from build123d import *


with BuildPart() as part:
    # Sketch1 → Revolve1 (revolve)
    with BuildSketch(Plane(origin=(0, 0, 0), x_dir=(0, 0, -1), z_dir=(1, 0, 0))):
        with BuildLine():
            Line((-10.35, -0.083114039), (-10.35, 2.416885961))
            add(Edge.make_bspline(
                [(-10.35, 2.416885961), (-10.35, 3.365522707), (-5.87405228, 4.241080394), (-2.867984372, 4.033812591), (-2.611626956, 4.324223727), (-2.731131844, 4.758475996), (-2.197387439, 5.360223564), (-0.492736408, 5.316885961), (0, 5.316885961)],
                knots=[0, 0, 0, 0, 0.734908426, 0.759492363, 0.786959078, 0.823764272, 0.867168962, 1, 1, 1, 1], degree=3))
            Line((0, 5.316885961), (0, 3.882124351))
            Line((0, 3.882124351), (-1.400856338, 3.882124351))
            Line((-1.400856338, 3.882124351), (-1.400856338, 2.565845829))
            Line((-1.400856338, 2.565845829), (-6.683387829, 1.648087396))
            Line((-6.683387829, 1.648087396), (-6.683387829, -4.921019872))
            Line((-6.683387829, -4.921019872), (-3.287892009, -7.171193847))
            Line((-3.287892009, -7.171193847), (-3.759677095, -7.883114039))
            Line((-3.759677095, -7.883114039), (-7.30583237, -5.533098981))
            Line((-7.30583237, -5.533098981), (-7.30583237, -7.883114039))
            Line((-7.30583237, -7.883114039), (-8.159470598, -7.883114039))
            Line((-8.159470598, -7.883114039), (-8.159470598, -7.762098691))
            Line((-8.159470598, -7.762098691), (-9.5, -4.383114039))
            Line((-9.5, -4.383114039), (-9.5, -2.883114039))
            Line((-9.5, -2.883114039), (-8, -2.883114039))
            Line((-8, -2.883114039), (-8, -2.583114039))
            Line((-8, -2.583114039), (-8.366666667, -2.216447373))
            Line((-8.366666667, -2.216447373), (-8, -1.849780706))
            Line((-8, -1.849780706), (-8.366666667, -1.483114039))
            Line((-8.366666667, -1.483114039), (-8, -1.116447373))
            Line((-8, -1.116447373), (-8.366666667, -0.749780706))
            Line((-8.366666667, -0.749780706), (-8, -0.383114039))
            Line((-8, -0.383114039), (-8, -0.083114039))
            Line((-8, -0.083114039), (-10.35, -0.083114039))
        make_face()
    revolve(axis=Axis((0, 6.890935363, 0), (0, -1, 0)))


solid = part.part
CAD build for the part. Positions are in the model's coordinates, mm. A direction names the side the tool comes from. Round coordinates to 2 decimals unless told otherwise and drop trailing zeros. Order: outer loops, then holes, each group sorted by start corner. A loop starts at its lowest first (then second) coordinate and runs counter-clockwise, first axis right, second up. Notation, with made-up numbers: (89.25, 38.25) -> (115.25, 38.25) arc R16 ccw to (115.25, 48.25) -> close; hole circle Ø10 at (22.25, -22). An arc over 180 degrees is marked (long way). Write each question's results on one line, items separated by ' | '.
1. Wall check: line 1 along Z through (x, y) = (0, -5.95); line 2 along X through (y, z) = (-6.8, 0); line 3 along X through (y, z) = (0.5, 0). Give the ranges that are in metal, low to high. Write a range as [from, to].
Findings below:
line 1: z = [-8.88, -7.31], [-6.68, -5.13], [5.13, 6.68], [7.31, 8.88] | line 2: x = [-8.54, -7.31], [-5.39, -3.85], [3.85, 5.39], [7.31, 8.54] | line 3: x = [-10.35, -6.68], [6.68, 10.35]
2. Cut at A-A (y = -6.75). Give the cut face in (x, z).
Findings below:
outline: circle Ø17.12 at (0, 0); circle Ø10.94 at (0, 0); hole circle Ø14.61 at (0, 0); hole circle Ø7.85 at (0, 0)
3. Flat gauge pins, fed straight in: P1, Ø5, axis at x = 1.5, z = -3.5, coming from the +Y side; P2, Ø5, axis at y = 0, z = 5, coming from the -X side; P3, Ø5.5, axis at x = 4, z = 2, coming from the +Y side. Where does each tip first touch, or does it go through?
Findings below:
P1: stops at y = 5.29 | P2: stops at x = -10.04 | P3: stops at y = 5.24
4. Pull direction Y, two halves, no side cores. Call faces 1 (the face through (4.445, -6.725, -5.798)), 2 (the face through (1.69, 2.51, -0.38)), 3 (the face through (8, -0.083, -3)), 4 (the face through (0, 3.882, 0)): pulls with the +Y half, pulls with the -Y half, needs draft (parallel to the pull), parting line crosses it, or undercut.
Findings below:
face 1: needs draft | face 2: undercut | face 3: undercut | face 4: pulls with the -Y half
5. 3-axis set-ups, long thin cutter, end or side, ignore diameter. For faces 5 (the face through (6.524, -1.682, -1.449)), 6 (the face through (6.3, 1.18, -8.21)), 7 (the face through (8.43, -3.62, 4.38)): which of +Z, -Z, +X, -X, +Y, -Y reach the whole face in a straight line?
Findings below:
face 5: none | face 6: +Y, -Y | face 7: -Y
